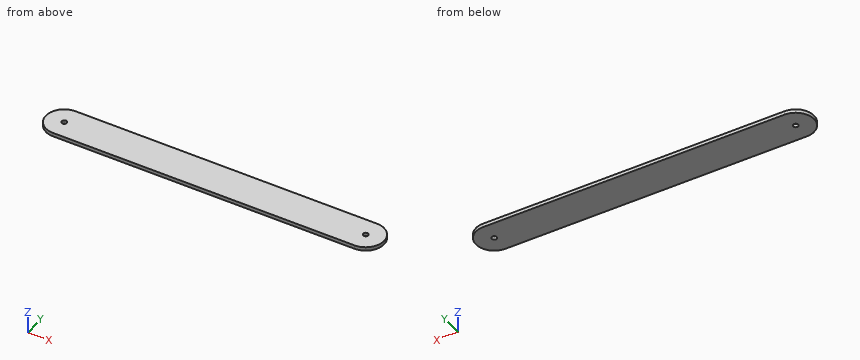
```python
from build123d import *

# Parameters (mm, degrees)
ESQUISSE1_R        = 2.1
BOSS_EXTRU_1_DEPTH = 3


with BuildPart() as part:
    # Esquisse1 → Boss.-Extru.1 (new body)
    with BuildSketch(Plane.XY):
        with BuildLine():
            Line((0, 15), (125, 15))
            ThreePointArc((125, 15), (140, 0), (125, -15))
            Line((125, -15), (0, -15))
            Line((0, -15), (0, 15))
        make_face()
        with Locations((125, 0)):
            Circle(ESQUISSE1_R, mode=Mode.SUBTRACT)
    extrude(amount=BOSS_EXTRU_1_DEPTH)

    # Symétrie1: part across plane


with BuildPart() as part_1:
    add(part.part)
    add(part.part.mirror(Plane(origin=(0, 15, 3), x_dir=(0, 0, 1), z_dir=(1, 0, 0))))


solid = part_1.part
```
Part model, mm, in its own coordinate system. Give positions to 0.01 mm unless a question says otherwise; leave off trailing zeros. Write each loop counter-clockwise with the first axis right and the second up, starting at its lowest first coordinate (ties: lowest second). Pieces come first, ordered by that corner, then holes. Notation, with made-up numbers: (-35.5, -23) -> (-24.5, -23) arc R26 ccw to (-24.5, -2) -> close; hole circle Ø4 at (83, 27.5). An arc over 180 degrees is marked (long way). Put each result on its own line as item: value. Start each with the question number.
Item 1: Cut at A-A (z = 2.2). List the corners of the cut face in (x, y), then the cut area to 3 significant figures.
Item 2: Wall check: L1, parallel to Y at x = 125, z = 1.45; L2, parallel to X at y = -13.5, z = 1.75; L3, parallel to X at y = -13, z = 1.9. Give the ranges that are in metal, low to high. Write a range as [from, to].
Item 3: Pin check, flat tips, straight feed: pin 1 Ø5 at (x, y) = (111.5, 2.5) entering from -Z; pin 2 Ø2.5 at (x, y) = (125, 0) entering from -Z. Stop position of each tip, or through.
Answer list:
1. outline: (-125, -15) -> (125, -15) arc R15 ccw to (125, 15) -> (-125, 15) arc R15 ccw to start; hole circle Ø4.2 at (-125, 0); hole circle Ø4.2 at (125, 0)
1. area: 8,180 mm2
2. L1: y = [-15, -2.1], [2.1, 15]
2. L2: x = [-131.54, 131.54]
2. L3: x = [-132.48, 132.48]
3. pin 1: stops at z = 0
3. pin 2: passes through
